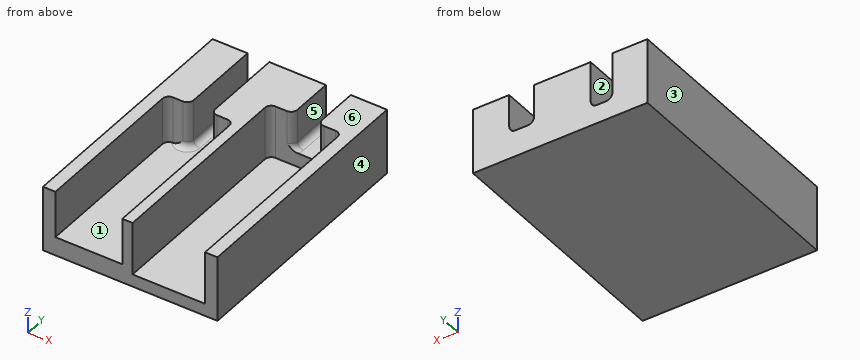
```python
from build123d import *

# Parameters (mm, degrees)
F0_W         = 3.5
F0_H         = 13.75
F0_W_2       = 4
F0_H_2       = 7.75
F1_DEPTH     = 2
F2_DEPTH     = 8.5
F3_DEPTH     = 1
F4_DEPTH     = 2.25
F5_R         = 1
F6_T1_DEPTH  = 12.75
F6_T3_DEPTH  = 6.75
F6_T6_ANGLE  = 233.2969892374
F6_T8_ANGLE  = 233.2969892374
F6_T12_ANGLE = 233.2969892374
F6_T17_ANGLE = 233.2969892374


# Not quite as in the source:
# - a fillet or chamfer that OpenCascade refuses, or shapes differently, is made with other operations: its cross-section is extruded or revolved along the edge and cut away or added


with BuildPart() as f1:
    # F0 (on Top) → F1 (new body)
    with BuildSketch(Plane.XY):
        Polygon((-12.025, -20), (-1.275, -20), (-1.275, 6.25), (-4.9, 6.25), (-8.4, 6.25), (-12.025, 6.25), align=None)
        Polygon((-14.025, -20), (-12.025, -20), (-12.025, 6.25), (-8.4, 6.25), (-8.4, 20), (-14.025, 20), align=None)
        Polygon((-1.275, -20), (0.375, -20), (0.375, 12.25), (4.2, 12.25), (4.2, 20), (-4.9, 20), (-4.9, 6.25), (-1.275, 6.25), align=None)
        with Locations((-6.65, 13.125)):
            Rectangle(F0_W, F0_H)
        with Locations((6.2, 16.125)):
            Rectangle(F0_W_2, F0_H_2)
        Polygon((0.375, -20), (12.025, -20), (12.025, 12.25), (8.2, 12.25), (4.2, 12.25), (0.375, 12.25), align=None)
        Polygon((12.025, -20), (14.025, -20), (14.025, 20), (8.2, 20), (8.2, 12.25), (12.025, 12.25), align=None)
    extrude(amount=-F1_DEPTH)

    # F0 (on Top) → F2 (join)
    with BuildSketch(Plane.XY):
        Polygon((-14.025, -20), (-12.025, -20), (-12.025, 6.25), (-8.4, 6.25), (-8.4, 20), (-14.025, 20), align=None)
        Polygon((-1.275, -20), (0.375, -20), (0.375, 12.25), (4.2, 12.25), (4.2, 20), (-4.9, 20), (-4.9, 6.25), (-1.275, 6.25), align=None)
        Polygon((12.025, -20), (14.025, -20), (14.025, 20), (8.2, 20), (8.2, 12.25), (12.025, 12.25), align=None)
    extrude(amount=F2_DEPTH)

    # F0 (on Top) → F3 (join)
    with BuildSketch(Plane.XY):
        Polygon((-12.025, -20), (-1.275, -20), (-1.275, 6.25), (-4.9, 6.25), (-8.4, 6.25), (-12.025, 6.25), align=None)
        with Locations((-6.65, 13.125)):
            Rectangle(F0_W, F0_H)
    extrude(amount=F3_DEPTH)

    # F0 (on Top) → F4 (join)
    with BuildSketch(Plane.XY):
        with Locations((6.2, 16.125)):
            Rectangle(F0_W_2, F0_H_2)
    extrude(amount=F4_DEPTH)

    # F5
    f5_edges = [f1.edges().sort_by_distance(p)[0] for p in [
        (-12.025, 6.25, 4.75),
        (-8.4, 6.25, 4.75),
        (-4.9, 6.25, 4.75),
        (-1.275, 6.25, 4.75),
        (4.2, 12.25, 5.375),
        (8.2, 12.25, 5.375),
        (0.375, 12.25, 4.25),
        (12.025, 12.25, 4.25),
    ]]
    fillet(f5_edges, radius=F5_R)

    # F6: fillet of radius 1 on 8 edges, made by hand

    # F6_s2 → F6_t1 (join)
    with BuildSketch(Plane.XZ.offset(-20)):
        with BuildLine():
            ThreePointArc((-8.4, 2), (-8.1071067812, 1.2928932188), (-7.4, 1))
            Line((-7.4, 1), (-8.4, 1))
            Line((-8.4, 1), (-8.4, 2))
        make_face()
        with BuildLine():
            ThreePointArc((-5.9, 1), (-5.1928932188, 1.2928932188), (-4.9, 2))
            Line((-4.9, 2), (-4.9, 1))
            Line((-4.9, 1), (-5.9, 1))
        make_face()
    extrude(amount=F6_T1_DEPTH)

    # F6_s4 → F6_t3 (join)
    with BuildSketch(Plane.XZ.offset(-20)):
        with BuildLine():
            ThreePointArc((5.2, 2.25), (4.4928932188, 2.5428932188), (4.2, 3.25))
            Line((4.2, 3.25), (4.2, 2.25))
            Line((4.2, 2.25), (5.2, 2.25))
        make_face()
        with BuildLine():
            ThreePointArc((8.2, 3.25), (7.9071067812, 2.5428932188), (7.2, 2.25))
            Line((7.2, 2.25), (8.2, 2.25))
            Line((8.2, 2.25), (8.2, 3.25))
        make_face()
    extrude(amount=F6_T3_DEPTH)

    # F6_s5 → F6_t6 (revolve)
    with BuildSketch(Plane(origin=(-2.5682338051, -1.9145124235, 0), x_dir=(0, 0, 1), z_dir=(0.8017442393, 0.5976672776, 0))):
        with BuildLine():
            ThreePointArc((1, -13.4307181447), (1.2928932188, -12.7236113635), (2, -12.4307181447))
            Line((2, -12.4307181447), (1, -12.4307181447))
            Line((1, -12.4307181447), (1, -13.4307181447))
        make_face()
    revolve(axis=Axis((-9.4, 7.25, 1), (0, 0, 1)), revolution_arc=F6_T6_ANGLE)

    # F6_s7 → F6_t8 (revolve)
    with BuildSketch(Plane(origin=(-5.9809240707, 4.4585323247, 0), x_dir=(0, 0, 1), z_dir=(-0.8017442393, 0.5976672776, 0))):
        with BuildLine():
            ThreePointArc((1, 5.4817433521), (1.2928932188, 4.774636571), (2, 4.4817433521))
            Line((2, 4.4817433521), (1, 4.4817433521))
            Line((1, 4.4817433521), (1, 5.4817433521))
        make_face()
    revolve(axis=Axis((-3.9, 7.25, 1), (0, 0, -1)), revolution_arc=F6_T8_ANGLE)


with BuildPart() as f6_tool10:
    # F6_s11 → F6_t12 (revolve)
    with BuildSketch(Plane(origin=(8.4060261742, 6.2663459654, 0), x_dir=(0, 0, 1), z_dir=(0.8017442393, 0.5976672776, 0))):
        with BuildLine():
            ThreePointArc((2.25, -10.7105758823), (2.5428932188, -10.0034691011), (3.25, -9.7105758823))
            Line((3.25, -9.7105758823), (2.25, -9.7105758823))
            Line((2.25, -9.7105758823), (2.25, -10.7105758823))
        make_face()
    revolve(axis=Axis((3.2, 13.25, 2.25), (0, 0, 1)), revolution_arc=F6_T12_ANGLE)

    split(bisect_by=Plane.XZ.offset(-12.25), keep=Keep.BOTTOM)


with BuildPart() as f1_1:
    add(f1.part)

    # F6_t9: union F6_tool10
    add(f6_tool10.part)


with BuildPart() as f6_tool15:
    # F6_s16 → F6_t17 (revolve)
    with BuildSketch(Plane(origin=(-0.4353827411, 0.3245598844, 0), x_dir=(0, 0, 1), z_dir=(-0.8017442393, 0.5976672776, 0))):
        with BuildLine():
            ThreePointArc((3.25, 17.1216501249), (2.5428932188, 17.4145433437), (2.25, 18.1216501249))
            Line((2.25, 18.1216501249), (2.25, 17.1216501249))
            Line((2.25, 17.1216501249), (3.25, 17.1216501249))
        make_face()
    revolve(axis=Axis((9.2, 13.25, 2.25), (0, 0, -1)), revolution_arc=F6_T17_ANGLE)

    split(bisect_by=Plane.XZ.offset(-12.25), keep=Keep.BOTTOM)


with BuildPart() as f1_2:
    add(f1_1.part)

    # F6_t14: union F6_tool15
    add(f6_tool15.part)


solid = f1_2.part
```
Model file for the job. Use its own axes, mm. Face numbers are marked on the shaded views. A direction names the side the tool comes from. Round coordinates to 2 decimals unless told otherwise and drop trailing zeros. Write each loop counter-clockwise with the first axis right and the second up, starting at its lowest first coordinate (ties: lowest second). Pieces come first, ordered by that corner, then holes. Notation, with made-up numbers: (72, 20.25) - (79, 20.25) arc R16 ccw to (79, 50.25) - close; hole circle Ø6 at (-10, 73). An arc over 180 degrees is marked (long way). One line per item, written item: value.
(1) Drop flat-ended pins along their axis: P1, Ø0.8, axis at x = -10, z = 3.5, coming from the -Y side; P2, Ø2, axis at x = 6, y = 16, coming from the +Z side. Give the stop position or say it passes through.
Values follow:
P1: stops at y = 6.25
P2: stops at z = 2.27
(2) Cut at B-B, the plane y = -5. Give the cut face in (x, z) (3 decimals), plus the area to 3 significant figures.
Values follow:
outline: (-14.025, -2) - (14.025, -2) - (14.025, 8.5) - (12.025, 8.5) - (12.025, 0) - (0.375, 0) - (0.375, 8.5) - (-1.275, 8.5) - (-1.275, 1) - (-12.025, 1) - (-12.025, 8.5) - (-14.025, 8.5) - close
area: 115 mm²
(3) Cut at A-A, the plane z = 7. Give the cut face in (x, y) (3 decimals).
Values follow:
outline: (-14.025, -20) - (-12.025, -20) - (-12.025, 5.25) arc R1 cw to (-11.025, 6.25) - (-9.4, 6.25) arc R1 ccw to (-8.4, 7.25) - (-8.4, 20) - (-14.025, 20) - close; (-4.9, 7.25) arc R1 ccw to (-3.9, 6.25) - (-2.275, 6.25) arc R1 cw to (-1.275, 5.25) - (-1.275, -20) - (0.375, -20) - (0.375, 11.25) arc R1 cw to (1.375, 12.25) - (3.2, 12.25) arc R1 ccw to (4.2, 13.25) - (4.2, 20) - (-4.9, 20) - close; (8.2, 13.25) arc R1 ccw to (9.2, 12.25) - (11.025, 12.25) arc R1 cw to (12.025, 11.25) - (12.025, -20) - (14.025, -20) - (14.025, 20) - (8.2, 20) - close
(4) Cut at C-C, the plane y = 14.5. Give the cut face in (x, z) (3 decimals).
Values follow:
outline: (-14.025, -2) - (14.025, -2) - (14.025, 8.5) - (8.2, 8.5) - (8.2, 3.25) arc R1 cw to (7.2, 2.25) - (5.2, 2.25) arc R1 cw to (4.2, 3.25) - (4.2, 8.5) - (-4.9, 8.5) - (-4.9, 2) arc R1 cw to (-5.9, 1) - (-7.4, 1) arc R1 cw to (-8.4, 2) - (-8.4, 8.5) - (-14.025, 8.5) - close
(5) 3-axis set-ups, long thin cutter, end or side, ignore diameter. For the marked faces 1, 2 and 3: which of +Z, -Z, +X, -X, +Y, -Y reach the whole face in a straight line?
Values follow:
face 1: +Z, -Y
face 2: +Z, +Y, -Y
face 3: +Z, -Z, -X, +Y, -Y
(6) Two-plate mould, pull along X, no slides. Class the marked faces 4, 5 and 6: pulls with the +X half, pulls with the -X half, needs draft (parallel to the pull), parting line crosses it, or undercut.
Values follow:
face 4: pulls with the +X half
face 5: undercut
face 6: needs draft
(7) Wall check: probe 1 along X at (y, z) = (-11, 2.5) (3 decimals); probe 2 along X at (y, z) = (18, 4.25) (3 decimals); probe 3 along Z at (x, y) = (4, -7). Give the ranges that are in metal, low to high.
Values follow:
probe 1: x = -14.025 to -12.025, -1.275 to 0.375, 12.025 to 14.025
probe 2: x = -14.025 to -8.4, -4.9 to 4.2, 8.2 to 14.025
probe 3: z = -2 to 0
